Geometry check sheet. Reference: the model listing, model coordinates, mm. Coordinates: 2 decimals unless noted, no trailing zeros. Loops run counter-clockwise (first coordinate to the right, second up) from the corner with the lowest first, then second, coordinate; pieces in that order, holes last. Notation, with made-up numbers: (11, 34.5) - (44, 34.5) arc R23 cw to (44, 71.5) - close; hole circle Ø11 at (-24, 78.25). An arc over 180 degrees is marked (long way). Write item = value, one per line. Start each with the question number.
Autodesk Inventor part; units mm, degrees
ref_plane "YZ Plane" through (0, 0, 0) normal (1, 0, 0) x (0, 1, 0)
ref_plane "XZ Plane" through (0, 0, 0) normal (0, 1, 0) x (-1, 0, 0)
ref_plane "XY Plane" through (0, 0, 0) normal (0, 0, 1) x (1, 0, 0)
sketch "Szkic1" plane through (0, 0, 0) normal (0, 1, 0) x (-1, 0, 0)
  circle A0 centre (45.7688, -11.3479) radius 1.5
  circle A1 centre (25.5188, -29.6192) radius 1.75
  circle A2 centre (66.0188, -29.6192) radius 1.75
  line L0 (-4.2312, -99.4192) -> (95.7688, -99.4192)
  line L1 (95.7688, -99.4192) -> (95.7688, -32.9192)
  line L2 (95.7688, -32.9192) -> (75.7688, -32.9192)
  line L3 (75.7688, -32.9192) -> (75.7688, -6.9192)
  line L4 (75.7688, -6.9192) -> (15.7688, -6.9192)
  line L5 (15.7688, -6.9192) -> (15.7688, -32.9192)
  line L6 (15.7688, -32.9192) -> (-4.2312, -32.9192)
  line L7 (-4.2312, -32.9192) -> (-4.2312, -99.4192)
  point P0 (0, 0)
  point P1 (0, 0)
extrude "Wyciągnięcie proste1" add sketch "Szkic1" along normal blind 2
sketch "Szkic2" plane through (0, 0, 0) normal (0, -1, 0) x (1, 0, 0)
  circle A0 centre (-1.3688, -61.7778) radius 1.5
  circle A1 centre (-21.5202, -42.1278) radius 1.5
  circle A2 centre (-70.0174, -42.1278) radius 1.5
  circle A3 centre (-90.1688, -61.7778) radius 1.5
  point P0 (0, 0)
extrude "Wyciągnięcie proste2" cut sketch "Szkic2" against normal blind 2
sketch "Szkic3" plane through (4.2312, 0, -32.9192) normal (1, 0, 0) x (0, 0, -1)
  line L0 (0, 0) -> (66.5, 0)
  line L1 (66.5, 0) -> (66.5, 2)
  line L2 (0, 2) -> (66.5, 2)
  line L3 (0, 0) -> (0, 2)
  line L4 (46.3508, 37) -> (66.9119, -1.4451)
  point P0 (-32.9192, 0)
  point P1 (65.0694, 2)
  point P2 (66.1391, 0)
extrude "Wyciągnięcie proste3" cut sketch "Szkic3" against normal through all contours L4 L2 L1 L0
sketch "Szkic4" plane through (0, 0, 0) normal (0, -1, 0) x (1, 0, 0)
  circle A0 centre (-11.7244, -89.168) radius 0.3048
  circle A1 centre (-14.2644, -89.168) radius 0.3048
  circle A2 centre (-14.2644, -86.628) radius 0.3048
  circle A3 centre (-11.7244, -86.628) radius 0.3048
  circle A4 centre (-80.1774, -89.676) radius 0.3048
  circle A5 centre (-77.6374, -89.676) radius 0.3048
  circle A6 centre (-77.6374, -87.136) radius 0.3048
  circle A7 centre (-80.1774, -87.136) radius 0.3048
  line L0 (-11.7244, -86.628) -> (-14.2644, -86.628)
  line L1 (-14.2644, -86.628) -> (-14.2644, -89.168)
  line L2 (-14.2644, -89.168) -> (-11.7244, -89.168)
  line L3 (-11.7244, -89.168) -> (-11.7244, -86.628)
  line L4 (-77.6374, -87.136) -> (-80.1774, -87.136)
  line L5 (-80.1774, -87.136) -> (-80.1774, -89.676)
  line L6 (-80.1774, -89.676) -> (-77.6374, -89.676)
  line L7 (-77.6374, -89.676) -> (-77.6374, -87.136)
  circle A8 centre (-78.9074, -88.406) radius 3.75
  circle A9 centre (-12.9944, -87.898) radius 3.75
  line L8 (-16.7444, -84.148) -> (-9.2444, -84.148)
  line L9 (-9.2444, -84.148) -> (-9.2444, -91.648)
  line L10 (-9.2444, -91.648) -> (-16.7444, -91.648)
  line L11 (-16.7444, -91.648) -> (-16.7444, -84.148)
  line L12 (-82.6574, -84.656) -> (-75.1574, -84.656)
  line L13 (-75.1574, -84.656) -> (-75.1574, -92.156)
  line L14 (-75.1574, -92.156) -> (-82.6574, -92.156)
  line L15 (-82.6574, -92.156) -> (-82.6574, -84.656)
  point P0 (0, 0)
  dimension "d6" = 7.5
  dimension "d7" = 7.5
extrude "Wyciągnięcie proste4" cut sketch "Szkic4" against normal through all contours A0 L2 L3 | L3 L2 A0 | A0 L2 A1 L1 A2 L0 A3 L3 | L3 L0 A3 | A3 L0 L3 | L2 L1 A1 | A1 L1 L2 | L0 L1 A2 | A2 L1 L0 | L6 L5 A4 | A4 L5 L6 | A4 L5 A7 L4 A6 L7 A5 L6 | L6 L7 A5 | A5 L7 L6 | L5 L4 A7 | A7 L4 L5 | L7 L4 A6 | A6 L4 L7 | A8 | L13 L14 A8 | A8 L12 L13 | A8 L15 L12 | L14 L15 A8 | A9 | L9 L10 A9 | A9 L8 L9 | A9 L11 L8 | L10 L11 A9
sketch "Szkic6" plane through (4.2312, 2, -32.9192) normal (1, 0, 0) x (0, 0, -1)
  line L0 (66.1391, -2) -> (65.0694, 0)
  line L1 (0, 0) -> (65.0694, 0)
  line L2 (0, -2) -> (0, 0)
  line L3 (66.1391, 0) -> (65, 0)
  line L4 (65, 0) -> (65, -3)
  line L5 (65, -3) -> (66.1391, -3)
  line L6 (66.1391, -3) -> (66.1391, 0)
  line L7 (0, -2) -> (66.1391, -2)
  point P0 (-32.9192, -2)
extrude "Wyciągnięcie proste6" add sketch "Szkic6" against normal blind 100 contours L0 L3 L6
properties part number "podstawa" material "Stal, węglowa"
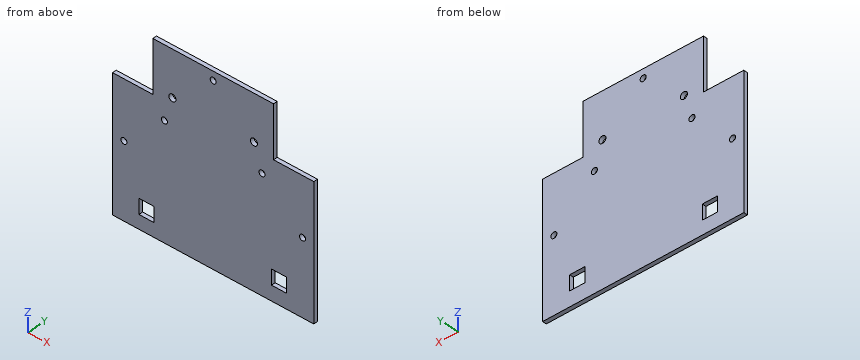
(1) Scan lines: line 1 (X direction, y = 0.45, z = -86); line 2 (Z direction, x = -90, y = 1.7); line 3 (Z direction, x = -66, y = 1.1). Record each from-to range of solid material in increasing order.
(2) Depth check by flat-ended pin: pin 1 (0.6 mm diameter, centred on x = -89, y = 0.5, fed in from +Z). Enter the tip coordinate at first touch or a pass-through.
(3) Sectioned sample at A-A on x = -77. Enter the section's corners in (y, z).
(4) Sectioned sample at B-B on y = 0.6. Count the separate pieces of the cut face and the enclosed holes in it, plus the area to 3 significant figures.
Working result:
q1.line_1 = -95.77 to -82.66, -75.16 to -16.74, -9.24 to 4.23
q1.line_2 = -99.06 to -63.27, -60.29 to -32.92
q1.line_3 = -99.06 to -31.37, -27.87 to -6.92
q2.pin_1 = -32.92
q3.outline = (0, -99.06) - (2, -99.06) - (2, -92.16) - (0, -92.16) - close; (0, -84.66) - (2, -84.66) - (2, -32.92) - (0, -32.92) - close
q4.separate_pieces = 1
q4.enclosed_holes = 9
q4.area = 8,010 mm2
